```python
from build123d import *

# Parameters (mm, degrees)
SKETCH1_W                      = 60
SKETCH1_H                      = 260
BASE_FLANGE1_DEPTH             = 2
EDGE_FLANGE1_STRIP_W           = 13
EDGE_FLANGE1_STRIP_H           = 2
EDGE_FLANGE1_STRIP_CUT_DEPTH   = 260
EDGE_FLANGE1_STRIP_2_W         = 13
EDGE_FLANGE1_STRIP_2_H         = 2
EDGE_FLANGE1_STRIP_CUT_2_DEPTH = 260
EDGE_FLANGE1_DEPTH             = 260
EDGE_FLANGE1_BEND_DEPTH        = 260
EDGE_FLANGE2_STRIP_W           = 13
EDGE_FLANGE2_STRIP_H           = 2
EDGE_FLANGE2_STRIP_CUT_DEPTH   = 260
EDGE_FLANGE2_STRIP_2_W         = 13
EDGE_FLANGE2_STRIP_2_H         = 2
EDGE_FLANGE2_STRIP_CUT_2_DEPTH = 260
EDGE_FLANGE2_DEPTH             = 260
EDGE_FLANGE2_BEND_DEPTH        = 260
SKETCH18_R                     = 5.5
CUT_EXTRUDE1_DEPTH             = 149.660687473


# Sheet-metal steps are written as plain solids
with BuildPart() as part:
    # Sketch1 → Base-Flange1 (new body)
    with BuildSketch(Plane.XY):
        Rectangle(SKETCH1_W, SKETCH1_H)
    extrude(amount=-BASE_FLANGE1_DEPTH)

    # Edge-Flange1 strip (across the edge) → Edge-Flange1 strip cut (cut)
    with BuildSketch(Plane(origin=(30, 130, -2), x_dir=(-1, 0, 0), z_dir=(0, -1, 0))):
        with Locations((-2, -1)):
            Rectangle(EDGE_FLANGE1_STRIP_W, EDGE_FLANGE1_STRIP_H)
    extrude(amount=EDGE_FLANGE1_STRIP_CUT_DEPTH, mode=Mode.SUBTRACT)

    # Edge-Flange1 strip 2 (across the edge) → Edge-Flange1 strip cut 2 (cut)
    with BuildSketch(Plane(origin=(-30, -130, -2), x_dir=(1, 0, 0), z_dir=(0, 1, 0))):
        with Locations((-2, -1)):
            Rectangle(EDGE_FLANGE1_STRIP_2_W, EDGE_FLANGE1_STRIP_2_H)
    extrude(amount=EDGE_FLANGE1_STRIP_CUT_2_DEPTH, mode=Mode.SUBTRACT)

    # Edge-Flange1 section (across the edge) → Edge-Flange1 (add)
    with BuildSketch(Plane(origin=(30, 130, -2), x_dir=(-1, 0, 0), z_dir=(0, -1, 0))):
        with BuildLine():
            Line((0, 2.5), (0, 38))
            Line((0, 38), (2, 38))
            Line((2, 38), (2, 2.5))
            ThreePointArc((2, 2.5), (2.732233047, 0.732233047), (4.5, 0))
            Line((4.5, 0), (4.5, -2))
            ThreePointArc((4.5, -2), (1.318019485, -0.681980515), (0, 2.5))
        make_face()
    extrude(amount=EDGE_FLANGE1_DEPTH)

    # Edge-Flange1 section 2 (across the edge) → Edge-Flange1 bend (add)
    with BuildSketch(Plane(origin=(-30, -130, -2), x_dir=(1, 0, 0), z_dir=(0, 1, 0))):
        with BuildLine():
            Line((0, 2.5), (0, 38))
            Line((0, 38), (2, 38))
            Line((2, 38), (2, 2.5))
            ThreePointArc((2, 2.5), (2.732233047, 0.732233047), (4.5, 0))
            Line((4.5, 0), (4.5, -2))
            ThreePointArc((4.5, -2), (1.318019485, -0.681980515), (0, 2.5))
        make_face()
    extrude(amount=EDGE_FLANGE1_BEND_DEPTH)

    # Edge-Flange2 strip (across the edge) → Edge-Flange2 strip cut (cut)
    with BuildSketch(Plane(origin=(28, 130, -40), x_dir=(0, 0, 1), z_dir=(0, -1, 0))):
        with Locations((-2, -1)):
            Rectangle(EDGE_FLANGE2_STRIP_W, EDGE_FLANGE2_STRIP_H)
    extrude(amount=EDGE_FLANGE2_STRIP_CUT_DEPTH, mode=Mode.SUBTRACT)

    # Edge-Flange2 strip 2 (across the edge) → Edge-Flange2 strip cut 2 (cut)
    with BuildSketch(Plane(origin=(-28, -130, -40), x_dir=(0, 0, 1), z_dir=(0, 1, 0))):
        with Locations((-2, -1)):
            Rectangle(EDGE_FLANGE2_STRIP_2_W, EDGE_FLANGE2_STRIP_2_H)
    extrude(amount=EDGE_FLANGE2_STRIP_CUT_2_DEPTH, mode=Mode.SUBTRACT)

    # Edge-Flange2 section (across the edge) → Edge-Flange2 (add)
    with BuildSketch(Plane(origin=(28, 130, -40), x_dir=(0, 0, 1), z_dir=(0, -1, 0))):
        with BuildLine():
            Line((0, 2.5), (0, 11))
            Line((0, 11), (2, 11))
            Line((2, 11), (2, 2.5))
            ThreePointArc((2, 2.5), (2.732233047, 0.732233047), (4.5, 0))
            Line((4.5, 0), (4.5, -2))
            ThreePointArc((4.5, -2), (1.318019485, -0.681980515), (0, 2.5))
        make_face()
    extrude(amount=EDGE_FLANGE2_DEPTH)

    # Edge-Flange2 section 2 (across the edge) → Edge-Flange2 bend (add)
    with BuildSketch(Plane(origin=(-28, -130, -40), x_dir=(0, 0, 1), z_dir=(0, 1, 0))):
        with BuildLine():
            Line((0, 2.5), (0, 11))
            Line((0, 11), (2, 11))
            Line((2, 11), (2, 2.5))
            ThreePointArc((2, 2.5), (2.732233047, 0.732233047), (4.5, 0))
            Line((4.5, 0), (4.5, -2))
            ThreePointArc((4.5, -2), (1.318019485, -0.681980515), (0, 2.5))
        make_face()
    extrude(amount=EDGE_FLANGE2_BEND_DEPTH)

    # Sketch18 → Cut-Extrude1 (cut, symmetric)
    with BuildSketch(Plane(origin=(30, 0, 0), x_dir=(0, 0, -1), z_dir=(1, 0, 0))):
        with Locations((20, -115)):
            Circle(SKETCH18_R)
        with Locations((20, -85)):
            Circle(SKETCH18_R)
    cut_extrude1 = extrude(amount=CUT_EXTRUDE1_DEPTH, both=True, mode=Mode.SUBTRACT)

    # Mirror1: Cut-Extrude1 across plane
    add(cut_extrude1.mirror(Plane.ZX), mode=Mode.SUBTRACT)


solid = part.part
```
Model file for the job. Use its own axes, mm. A direction names the side the tool comes from. Coordinates: 2 decimals unless noted, no trailing zeros. Order: outer loops, then holes, each group sorted by start corner. A loop starts at its lowest first (then second) coordinate and runs counter-clockwise, first axis right, second up. Notation, with made-up numbers: (3.5, 40) - (34.5, 40) arc R23 ccw to (34.5, 65) - close; hole circle Ø6 at (11, -20). An arc over 180 degrees is marked (long way). Return JSON: item names as keys, results as strings. Group by question number.
1) Saw through at C-C, the plane y = 70.5. Write the cut outline in (x, z), plus the area to 3 significant figures.
2) Flat gauge pins, fed straight in: P1, Ø2.5, axis at x = -23, y = 60, coming from the +Z side; P2, Ø2, axis at y = 18.5, z = -39, coming from the +X side; P3, Ø4, axis at x = 9.5, y = -0.5, coming from the -Z side; P4, Ø1, axis at y = 33, z = -39.5, coming from the -X side. Where does each tip first touch, or does it go through?
3) Probe line 1 (Y direction, x = -29.4, z = -20); line 2 (X direction, y = -90, z = -28); line 3 (Z direction, x = -1.5, y = 68.5). List the from-to ranges inside material, lowest first. Write a range as from..to.
4) Saw through at A-A, the plane y = -85. Write the cut outline in (x, z).
5) Tool access for faces 1 (the cylindrical face through (-28.986, 79.547, -19.284)), 2 (the flat face through (28, 2, -20)): list every direction of +Z, -Z, +X, -X, +Y, -Y with a clear straight run to the whole face (end or side of a thin tool).
6) Saw through at D-D, the plane z = -20. Count the separate pieces of the cut face and the enclosed holes in it, plus the area to 3 significant figures.
7) Saw through at B-B, the plane x = 22. Write the cut outline in (y, z).
8) Mould opens along X. For faces 3 (the flat face through (21, 2, -38)), 4 (the flat face through (0, 2, 0)), 5 (the flat face through (-30, -2, -20)) say: released by +X, released by -X, zero draft, split by the parting line, or undercut.
Values found:
{
 "1": {"outline": "(-30, -35.5) arc R4.5 ccw to (-25.5, -40) - (-17, -40) - (-17, -38) - (-25.5, -38) arc R2.5 cw to (-28, -35.5) - (-28, -4.5) arc R2.5 cw to (-25.5, -2) - (25.5, -2) arc R2.5 cw to (28, -4.5) - (28, -35.5) arc R2.5 cw to (25.5, -38) - (17, -38) - (17, -40) - (25.5, -40) arc R4.5 ccw to (30, -35.5) - (30, -4.5) arc R4.5 ccw to (25.5, 0) - (-25.5, 0) arc R4.5 ccw to (-30, -4.5) - close", "area": "304 mm²"},
 "2": {"P1": "stops at z = 0", "P2": "stops at x = 29.24", "P3": "stops at z = -2", "P4": "stops at x = -28.33"},
 "3": {"line 1": "y = -130..-120.5, -109.5..-90.5, -79.5..79.5, 90.5..109.5, 120.5..130", "line 2": "x = -30..-28, 28..30", "line 3": "z = -2..0"},
 "4": {"outline": "(-30, -35.5) arc R4.5 ccw to (-25.5, -40) - (-17, -40) - (-17, -38) - (-25.5, -38) arc R2.5 cw to (-28, -35.5) - (-28, -25.5) - (-30, -25.5) - close; (-30, -14.5) - (-28, -14.5) - (-28, -4.5) arc R2.5 cw to (-25.5, -2) - (25.5, -2) arc R2.5 cw to (28, -4.5) - (28, -14.5) - (30, -14.5) - (30, -4.5) arc R4.5 ccw to (25.5, 0) - (-25.5, 0) arc R4.5 ccw to (-30, -4.5) - close; (17, -40) - (25.5, -40) arc R4.5 ccw to (30, -35.5) - (30, -25.5) - (28, -25.5) - (28, -35.5) arc R2.5 cw to (25.5, -38) - (17, -38) - close"},
 "5": {"face 1": "+X, -X", "face 2": "+Y, -Y"},
 "6": {"separate pieces": "10", "enclosed holes": "0", "area": "864 mm²"},
 "7": {"outline": "(-130, -40) - (130, -40) - (130, -38) - (-130, -38) - close; (-130, -2) - (130, -2) - (130, 0) - (-130, 0) - close"},
 "8": {"face 3": "undercut", "face 4": "zero draft", "face 5": "released by -X"}
}
